Can you work these out from the model? Positions are in its coordinate system, mm. Coordinates: 2 decimals unless noted, no trailing zeros. Loops run counter-clockwise (first coordinate to the right, second up) from the corner with the lowest first, then second, coordinate; pieces in that order, holes last. Notation, with made-up numbers: M -29,-22 L 13,-22 A24 cw 13,0 Z; hole C -8.75,77 d7. An arc over 180 degrees is marked long. Answer as a JSON object with one key per item and string values. Group by question number.
Item 1: We'd pull the mould along Z, two halves only. Please class faces 1 (the flat face through (-4, 1.27, 0)), 2 (the cylindrical face through (3.85, 0.63, 17.36)), 3 (the cylindrical face through (4.377, 0.626, -12.11)): +Z half, -Z half, draft (parallel to the pull), parting line (faces both ways), or undercut.
Item 2: I'm going to push a flat-ended pin straight in: pin 1 Ø2 at (x, z) = (-3.4, 11.79) entering from +Y. Where does the tip first touch, or does it pass through?
Item 3: Suppose I cut it at A-A (z = 0). Write out the boundary of the cut face in (x, y) (1 decimal), then the cut area to 3 significant figures.
Item 4: Suppose I cut it at B-B (x = 0). Write out the boundary of the cut face in (y, z) (3 decimals), then the cut area to 3 significant figures.
Item 5: If I drill on line 1 (Z direction, x = -13, y = 1.15); line 2 (Z direction, x = -12.5, y = 0.2); line 3 (X direction, y = 0.7, z = 4), over which ranges is the centre line in solid material (lowest first)?
Item 6: Suppose I cut it at D-D (y = 1.05). Count the separate pieces of the cut face and the enclosed holes in it, then the cut area to 3 significant figures.
Item 7: Suppose I cut it at C-C (z = 5). Write out the boundary of the cut face in (x, y).
Autodesk Inventor part; units mm, degrees
ref_plane "YZ Plane" through (0, 0, 0) normal (1, 0, 0) x (0, 1, 0)
ref_plane "XZ Plane" through (0, 0, 0) normal (0, 1, 0) x (-1, 0, 0)
ref_plane "XY Plane" through (0, 0, 0) normal (0, 0, 1) x (1, 0, 0)
sketch "Sketch1" plane through (0, 0, 0) normal (0, 1, 0) x (-1, 0, 0)
  circle A0 centre (0, 0) radius 17.78
  dimension "d0" = 35.56
extrude "Extrusion1" add sketch "Sketch1" along normal blind 1.27
sketch "Sketch2" plane through (0, 1.27, 0) normal (0, 1, 0) x (1, 0, 0)
  circle A0 centre (0, 0) radius 17.78
hole "Hole1" at (0, 1.27, 0) direction (0, -1, 0) diameter 6.35 end through all
sketch "Sketch3" plane through (0, 1.27, 0) normal (0, 1, 0) x (1, 0, 0)
  line L0 (0, 0) -> (-13.6144, 0)
  dimension "d10" = 13.6144
hole "Hole2" at (-13.6144, 1.27, 0) direction (0, -1, 0) diameter 4.9022 end through all
pattern_circular "Circular Pattern1" count 3 over 360 about axis through (0, -49.0355, 0) along (0, 1, 0) of "Hole2"
sketch "Sketch5" plane through (0, 1.27, 0) normal (0, 1, 0) x (1, 0, 0)
  circle A0 centre (-13.6144, 0) radius 2.4511
  circle A1 centre (6.8072, 11.7904) radius 2.4511
  line L0 (-13.6144, 0) -> (6.8072, 11.7904)
  circle A2 centre (6.8072, -11.7904) radius 2.4511
  line L1 (6.8072, 11.7904) -> (6.8072, -11.7904)
  line L2 (6.8072, -11.7904) -> (-13.6144, 0)
  line L3 (-13.6144, 0) -> (-13.6144, -11.7904)
  line L4 (-13.6144, -11.7904) -> (6.8072, -11.7904)
  line L5 (-13.6144, 0) -> (-13.6144, 11.7904)
  line L6 (-13.6144, 11.7904) -> (6.8072, 11.7904)
  circle A3 centre (-3.4036, 11.7904) radius 0.635
  circle A4 centre (-3.4036, -11.7904) radius 0.635
  point P0 (0, 0)
  dimension "d28" = 1.27
hole "Hole4" at (-3.4036, 1.27, 11.7904) at (-3.4036, 1.27, -11.7904) direction (0, -1, 0) diameter 1.905 depth 6.35 tip angle 118
sketch "Sketch6" plane through (0, 1.27, 0) normal (0, 1, 0) x (1, 0, 0)
  circle A0 centre (6.8072, 11.7904) radius 2.4511
  circle A1 centre (6.8072, -11.7904) radius 2.4511
  line L0 (6.8072, 11.7904) -> (6.8072, -11.7904)
  line L1 (0, 0) -> (17.6436, 0)
  line L2 (0, 0) -> (12.7, 0)
  line L3 (0, 0) -> (17.78, 0)
  circle A2 centre (0, 0) radius 17.78
  line L4 (6.8072, 0) -> (10.6172, 0)
  line L5 (10.6172, 0) -> (10.6172, 6.35)
  line L6 (10.6172, 6.35) -> (10.6172, -6.35)
  line L7 (10.6172, -6.35) -> (10.6172, -3.175)
  line L8 (10.6172, -3.175) -> (10.6172, 3.175)
  line L9 (10.6172, 6.35) -> (10.6172, 3.175)
  line L10 (10.6172, -3.175) -> (10.6172, -6.35)
  circle A3 centre (10.6172, 4.7625) radius 3.175
  circle A4 centre (10.6172, -4.7625) radius 3.175
  dimension "d36" = 12.7
  dimension "d37" = 3.81
  dimension "d38" = 6.35
  dimension "d39" = 12.7
  dimension "d40" = 3.175
  dimension "d41" = 6.35
  dimension "d42" = 180
  dimension "d43" = 6.35
  dimension "d44" = 6.35
hole "Hole5" at (10.6172, 1.27, -4.7625) at (10.6172, 1.27, 4.7625) direction (0, -1, 0) diameter 6.35 depth 6.35
properties part number "buffer" material "PBT Plastic"
From the geometry:
{
 "1": {"face 1": "draft", "face 2": "parting line", "face 3": "undercut"},
 "2": {"pin 1": "y = 1.27"},
 "3": {"outline": "M -17.8,0 L -16.1,0 L -16.1,1.3 L -17.8,1.3 Z; M -11.2,0 L -3.2,0 L -3.2,1.3 L -11.2,1.3 Z; M 3.2,0 L 17.8,0 L 17.8,1.3 L 3.2,1.3 Z", "area": "30.9 mm2"},
 "4": {"outline": "M 0,-17.78 L 1.27,-17.78 L 1.27,-3.175 L 0,-3.175 Z; M 0,3.175 L 1.27,3.175 L 1.27,17.78 L 0,17.78 Z", "area": "37.1 mm2"},
 "5": {"line 1": "-12.13 to -2.37, 2.37 to 12.13", "line 2": "-12.64 to -2.18, 2.18 to 12.64", "line 3": "-17.32 to 7.54, 13.7 to 17.32"},
 "6": {"separate pieces": "1", "enclosed holes": "8", "area": "836 mm2"},
 "7": {"outline": "M -17.06,0 L 7.45,0 L 7.45,1.27 L -17.06,1.27 Z; M 13.78,0 L 17.06,0 L 17.06,1.27 L 13.78,1.27 Z"}
}
